CAD build for the part. Positions are in the model's coordinates, mm. Face numbers are marked on the shaded views. A direction names the side the tool comes from. Round coordinates to 2 decimals unless told otherwise and drop trailing zeros. Loops run counter-clockwise (first coordinate to the right, second up) from the corner with the lowest first, then second, coordinate; pieces in that order, holes last.
from build123d import *

# Parameters (mm, degrees)
SKETCH1_W               = 70
SKETCH1_H               = 30
BOSS_EXTRUDE1_DEPTH     = 10
SKETCH2_R               = 20
BOSS_EXTRUDE2_DEPTH     = 10
CUT_EXTRUDE1_DEPTH      = 42.533119315
CUT_EXTRUDE1_DEPTH_BACK = 42.533119315
SKETCH3_R               = 15
CUT_EXTRUDE2_DEPTH      = 42.533119315
CUT_EXTRUDE2_DEPTH_BACK = 42.533119315
SKETCH4_R               = 1.6
FILLET1_R               = 5


with BuildPart() as part:
    # Sketch1 → Boss-Extrude1 (new body)
    with BuildSketch(Plane(origin=(0, 0, 0), x_dir=(1, 0, 0), z_dir=(0, 1, 0))):
        Rectangle(SKETCH1_W, SKETCH1_H)
    extrude(amount=BOSS_EXTRUDE1_DEPTH)

    # Sketch2 → Boss-Extrude2 (add)
    with BuildSketch(Plane(origin=(0, 0, 0), x_dir=(1, 0, 0), z_dir=(0, 1, 0))):
        Circle(SKETCH2_R)
    extrude(amount=BOSS_EXTRUDE2_DEPTH)

    # Sketch3 → Cut-Extrude1 (cut, two sides: drawn at the far end of the back side and taken through both)
    with BuildSketch(Plane(origin=(0, 10, 0), x_dir=(1, 0, 0), z_dir=(0, 1, 0)).offset(-CUT_EXTRUDE1_DEPTH_BACK)):
        with Locations(Location((0, 0, 0), (0, 0, 270))):
            Circle(SKETCH3_R)
    extrude(amount=CUT_EXTRUDE1_DEPTH + CUT_EXTRUDE1_DEPTH_BACK, mode=Mode.SUBTRACT)

    # Sketch4 → Cut-Extrude2 (cut, two sides: drawn at the far end of the back side and taken through both)
    with BuildSketch(Plane(origin=(0, 10, 0), x_dir=(1, 0, 0), z_dir=(0, 1, 0)).offset(-CUT_EXTRUDE2_DEPTH_BACK)):
        with Locations(Location((-30, 10, 0), (0, 0, 270))):
            Circle(SKETCH4_R)
        with Locations(Location((30, -10, 0), (0, 0, 270))):
            Circle(SKETCH4_R)
        with Locations(Location((30, 10, 0), (0, 0, 270))):
            Circle(SKETCH4_R)
        with Locations(Location((-30, -10, 0), (0, 0, 270))):
            Circle(SKETCH4_R)
    extrude(amount=CUT_EXTRUDE2_DEPTH + CUT_EXTRUDE2_DEPTH_BACK, mode=Mode.SUBTRACT)

    # Fillet1
    fillet1_edges = [part.edges().sort_by_distance(p)[0] for p in [
        (-13.228756555, 5, -15),
        (13.228756555, 5, -15),
        (13.228756555, 5, 15),
        (-13.228756555, 5, 15),
        (35, 5, 15),
        (-35, 5, 15),
        (-35, 5, -15),
        (35, 5, -15),
    ]]
    fillet(fillet1_edges, radius=FILLET1_R)


solid = part.part
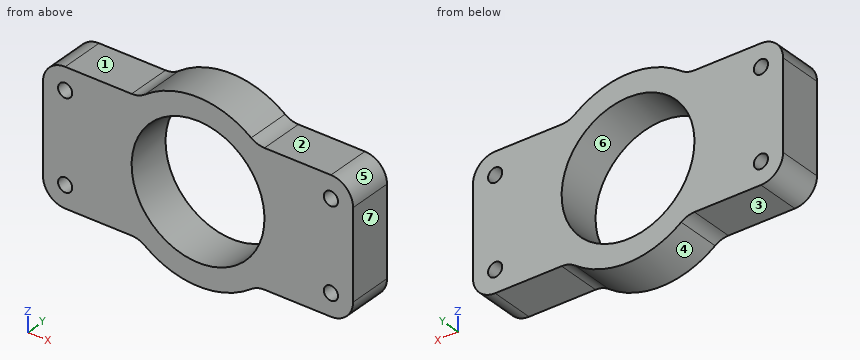
Item 1: Wall check: L1, parallel to Z at x = -30, y = 8; L2, parallel to Z at x = 0, y = 6.5; L3, parallel to X at y = 7.25, z = -10. Give the ranges that are in metal, low to high.
Verdict:
L1: z = -15 to -11.6, -8.4 to 8.4, 11.6 to 15
L2: z = -20 to -15, 15 to 20
L3: x = -35 to -31.6, -28.4 to -11.18, 11.18 to 28.4, 31.6 to 35
Item 2: Cut at A-A (z = 0). List the corners of the cut face in (x, y), plus the area to 3 significant figures.
Verdict:
outline: (-35, 0) - (-15, 0) - (-15, 10) - (-35, 10) - close; (15, 0) - (35, 0) - (35, 10) - (15, 10) - close
area: 400 mm2
Item 3: 3-axis set-ups, long thin cutter, end or side, ignore diameter. For the marked faces 1, 2 and 3: which of +Z, -Z, +X, -X, +Y, -Y reach the whole face in a straight line?
Verdict:
face 1: +Z, -X, +Y, -Y
face 2: +Z, +X, +Y, -Y
face 3: -Z, -X, +Y, -Y
Item 4: Flat gauge pins, fed straight in: P1, Ø1, axis at y = 3, z = -13.5, coming from the +X side; P2, Ø4, axis at x = -21.5, y = 8, coming from the -Z side; P3, Ø3, axis at x = -21.5, y = 7, coming from the +Z side. Where does each tip first touch, or does it go through?
Verdict:
P1: stops at x = 34
P2: stops at z = -15
P3: stops at z = 15
Item 5: Mould opens along Z. For the marked faces 4, 5, 6 and 7 say: released by +Z, released by -Z, zero draft, split by the parting line, or undercut.
Verdict:
face 4: released by -Z
face 5: released by +Z
face 6: undercut
face 7: zero draft
Item 6: Cut at C-C (x = -4.5). List the corners of the cut face in (y, z), plus the area to 3 significant figures.
Verdict:
outline: (0, -19.49) - (10, -19.49) - (10, -14.31) - (0, -14.31) - close; (0, 14.31) - (10, 14.31) - (10, 19.49) - (0, 19.49) - close
area: 104 mm2
Item 7: Cut at D-D (x = -18). List the corners of the cut face in (y, z).
Verdict:
outline: (0, -15) - (10, -15) - (10, 15) - (0, 15) - close
Item 8: Cut at B-B (y = 6.25). List the corners of the cut face in (x, z), plus the area to 3 significant figures.
Verdict:
outline: (-35, -10) arc R5 ccw to (-30, -15) - (-15, -15) arc R5 cw to (-12, -16) arc R20 ccw to (12, -16) arc R5 cw to (15, -15) - (30, -15) arc R5 ccw to (35, -10) - (35, 10) arc R5 ccw to (30, 15) - (15, 15) arc R5 cw to (12, 16) arc R20 ccw to (-12, 16) arc R5 cw to (-15, 15) - (-30, 15) arc R5 ccw to (-35, 10) - close; hole circle Ø3.2 at (-30, -10); hole circle Ø3.2 at (-30, 10); hole circle Ø30 at (0, 0); hole circle Ø3.2 at (30, -10); hole circle Ø3.2 at (30, 10)
area: 1,520 mm2
